from build123d import *

# Parameters (mm, degrees)
SKETCH1_R           = 125
BOSS_EXTRUDE1_DEPTH = 20
CUT_EXTRUDE1_DEPTH  = 21


with BuildPart() as part:
    # Sketch1 → Boss-Extrude1 (new body)
    with BuildSketch(Plane.XY):
        Circle(SKETCH1_R)
    extrude(amount=BOSS_EXTRUDE1_DEPTH)

    # Sketch2 → Cut-Extrude1 (cut, through all)
    with BuildSketch(Plane.XY.offset(20)):
        with BuildLine():
            Line((-9.682458366, 2.5), (-15, 2.5))
            Line((-15, 2.5), (-15, -2.5))
            Line((-15, -2.5), (-9.682458366, -2.5))
            ThreePointArc((-9.682458366, -2.5), (10, 0), (-9.682458366, 2.5))
        make_face()
    extrude(amount=-CUT_EXTRUDE1_DEPTH, mode=Mode.SUBTRACT)


solid = part.part
Here's how the part is built. I have some questions about the finished solid (model axes, mm). A direction names the side the tool comes from. Round coordinates to 2 decimals unless told otherwise and drop trailing zeros. Loops run counter-clockwise (first coordinate to the right, second up) from the corner with the lowest first, then second, coordinate; pieces in that order, holes last. Notation, with made-up numbers: (63.5, 59) - (77.5, 59) arc R25 cw to (77.5, 87) - close; hole circle Ø8 at (-9.5, 88.25). An arc over 180 degrees is marked (long way). One line per question, with ' | ' between items. Start each with the question number.
Q1. Will these pins go through, and if not, where does the flat tip stop? pin 1 (6 mm diameter, centred on x = -13.5, z = 6.5, fed in from +Y); pin 2 (12 mm diameter, centred on y = -73, z = 4.5, fed in from +X); pin 3 (6 mm diameter, centred on x = -86, z = 9, fed in from -Y).
Q2. I want a section at B-B (z = 3). Write out the boundary of the cut face in (x, y).
Q3. I want a section at A-A (x = 0). Write out the boundary of the cut face in (y, z), then the cut area to 3 significant figures.
Q4. I want a section at C-C (x = -75). Write out the boundary of the cut face in (y, z).
Q5. Please list where these lines run through material, in increasing order: line 1 (Y direction, x = 0, z = 15.75); line 2 (X direction, y = -0.5, z = 11.75); line 3 (Y direction, x = -11.5, z = 19.25). Write a range as [from, to].
Q6. We'd pull the mould along Y, two halves only. Please class faces 3 (the flat face through (-2, -26, 20)), 4 (the cylindrical face through (10, 0, 10)), 5 (the cylindrical face through (-124.88, 5.5, 9.86)): +Y half, -Y half, draft (parallel to the pull), parting line (faces both ways), or undercut.
Q7. I want a section at D-D (y = -92). Write out the boundary of the cut face in (x, z).
Q8. For faces 1 (the flat face through (-12, -2.5, 10)), 2 (the flat face through (-2, -26, 0)), which set-ups out of +Z, -Z, +X, -X, +Y, -Y let a thin tool reach every point of the face, with its end or its side?
Response values:
1) pin 1: stops at y = 124.56 | pin 2: stops at x = 105.53 | pin 3: stops at y = -93.47
2) outline: circle Ø250 at (0, 0); hole (-15, -2.5) - (-9.68, -2.5) arc R10 ccw (long way) to (-9.68, 2.5) - (-15, 2.5) - close
3) outline: (-125, 0) - (-10, 0) - (-10, 20) - (-125, 20) - close; (10, 0) - (125, 0) - (125, 20) - (10, 20) - close | area: 4,600 mm²
4) outline: (-100, 0) - (100, 0) - (100, 20) - (-100, 20) - close
5) line 1: y = [-125, -10], [10, 125] | line 2: x = [-125, -15], [9.99, 125] | line 3: y = [-124.47, -2.5], [2.5, 124.47]
6) face 3: draft | face 4: undercut | face 5: parting line
7) outline: (-84.62, 0) - (84.62, 0) - (84.62, 20) - (-84.62, 20) - close
8) face 1: +Z, -Z | face 2: -Z, +X, -X, +Y, -Y
